from build123d import *

# Parameters (mm, degrees)
SKETCH1_W           = 100
SKETCH1_H           = 80
BOSS_EXTRUDE1_DEPTH = 4
SKETCH2_R           = 1
CUT_EXTRUDE1_DEPTH  = 65.156059729
BOSS_EXTRUDE2_DEPTH = 4
SKETCH4_R           = 1
CUT_EXTRUDE2_DEPTH  = 4
SKETCH5_R           = 1
CUT_EXTRUDE3_DEPTH  = 4
SKETCH6_R           = 6
CUT_EXTRUDE4_DEPTH  = 95.424573073
BOSS_EXTRUDE3_DEPTH = 4
SKETCH8_R           = 2.75
CUT_EXTRUDE5_DEPTH  = 308.949597178
CUT_EXTRUDE6_DEPTH  = 308.949597178
SKETCH11_R          = 1
SKETCH11_R_2        = 6
SKETCH11_W          = 15
SKETCH11_H          = 40
CUT_EXTRUDE7_DEPTH  = 4
SKETCH14_R          = 1
SKETCH14_R_2        = 6
BOSS_EXTRUDE5_DEPTH = 4
SKETCH15_R          = 6
CUT_EXTRUDE8_DEPTH  = 256.598728949
FILLET1_R           = 50


with BuildPart() as part:
    # Sketch1 → Boss-Extrude1 (new body)
    with BuildSketch(Plane(origin=(0, 0, 0), x_dir=(1, 0, 0), z_dir=(0, 1, 0))):
        Rectangle(SKETCH1_W, SKETCH1_H)
    extrude(amount=BOSS_EXTRUDE1_DEPTH)

    # Sketch2 → Cut-Extrude1 (cut, through all)
    with BuildSketch(Plane(origin=(0, 4, 0), x_dir=(1, 0, 0), z_dir=(0, 1, 0))):
        with Locations(Location((-40, 30, 0), (0, 0, 270))):
            Circle(SKETCH2_R)
        with Locations(Location((16.7, 30, 0), (0, 0, 270))):
            Circle(SKETCH2_R)
        with Locations(Location((16.7, -17.9, 0), (0, 0, 270))):
            Circle(SKETCH2_R)
        with Locations(Location((-40, -17.9, 0), (0, 0, 270))):
            Circle(SKETCH2_R)
    extrude(amount=-CUT_EXTRUDE1_DEPTH, mode=Mode.SUBTRACT)

    # Sketch3 → Boss-Extrude2 (add)
    with BuildSketch(Plane(origin=(0, 4, 0), x_dir=(1, 0, 0), z_dir=(0, 1, 0))):
        Polygon((7.993464363, -40), (50, -40), (50, -80), (-50, -80), (-50, -40), (-32.006535637, -40), (-32.006535637, -55), (7.993464363, -55), align=None)
    extrude(amount=-BOSS_EXTRUDE2_DEPTH)

    # Sketch4 → Cut-Extrude2 (cut)
    with BuildSketch(Plane(origin=(0, 4, 0), x_dir=(1, 0, 0), z_dir=(0, 1, 0))):
        with Locations(Location((-22.506535637, -61.25, 0), (0, 0, 270))):
            Circle(SKETCH4_R)
        with Locations(Location((-22.506535637, -73.75, 0), (0, 0, 270))):
            Circle(SKETCH4_R)
        with Locations(Location((-1.506535637, -73.75, 0), (0, 0, 270))):
            Circle(SKETCH4_R)
        with Locations(Location((-1.506535637, -61.25, 0), (0, 0, 270))):
            Circle(SKETCH4_R)
    extrude(amount=-CUT_EXTRUDE2_DEPTH, mode=Mode.SUBTRACT)

    # Sketch5 → Cut-Extrude3 (cut)
    with BuildSketch(Plane(origin=(0, 4, 0), x_dir=(1, 0, 0), z_dir=(0, 1, 0))):
        with Locations(Location((30, -45, 0), (0, 0, 270))):
            Circle(SKETCH5_R)
        with Locations(Location((30, -70, 0), (0, 0, 270))):
            Circle(SKETCH5_R)
    extrude(amount=-CUT_EXTRUDE3_DEPTH, mode=Mode.SUBTRACT)

    # Sketch6 → Cut-Extrude4 (cut, through all)
    with BuildSketch(Plane(origin=(0, 4, 0), x_dir=(1, 0, 0), z_dir=(0, 1, 0))):
        with Locations(Location((-12.006535637, -31, 0), (0, 0, 270))):
            Circle(SKETCH6_R)
    extrude(amount=-CUT_EXTRUDE4_DEPTH, mode=Mode.SUBTRACT)

    # Sketch7 → Boss-Extrude3 (add)
    with BuildSketch(Plane.XZ):
        with BuildLine():
            Line((-146.240473223, -40), (-50, -40))
            Line((-50, -40), (-50, 80))
            Line((-50, 80), (50, 80))
            Line((50, 80), (50, -40))
            Line((50, -40), (122.22740195, -40))
            ThreePointArc((122.22740195, -40), (148.208164063, -25), (148.208164063, 5))
            Line((148.208164063, 5), (13.974226477, 237.5))
            ThreePointArc((13.974226477, 237.5), (-12.006535637, 252.5), (-37.98729775, 237.5))
            Line((-37.98729775, 237.5), (-172.221235337, 5))
            ThreePointArc((-172.221235337, 5), (-172.221235337, -25), (-146.240473223, -40))
        make_face()
    extrude(amount=-BOSS_EXTRUDE3_DEPTH)

    # Sketch8 → Cut-Extrude5 (cut, through all)
    with BuildSketch(Plane.XZ):
        with Locations(Location((-27.006535637, -20.35, 0), (0, 0, 270))):
            Circle(SKETCH8_R)
        with Locations(Location((2.993464363, -20.35, 0), (0, 0, 270))):
            Circle(SKETCH8_R)
        with Locations(Location((-80.586867359, 124.415381057, 0), (0, 0, 90))):
            Circle(SKETCH8_R)
        with Locations(Location((-95.586867359, 98.434618943, 0), (0, 0, 90))):
            Circle(SKETCH8_R)
        with Locations(Location((71.573796086, 98.434618943, 0), (0, 0, 90))):
            Circle(SKETCH8_R)
        with Locations(Location((56.573796086, 124.415381057, 0), (0, 0, 90))):
            Circle(SKETCH8_R)
    extrude(amount=-CUT_EXTRUDE5_DEPTH, mode=Mode.SUBTRACT)

    # Sketch9 → Cut-Extrude6 (cut, through all)
    with BuildSketch(Plane(origin=(0, 4, 0), x_dir=(1, 0, 0), z_dir=(0, 1, 0))):
        with BuildLine():
            Line((32.993464363, -204.557713659), (-57.006535637, -204.557713659))
            Line((-57.006535637, -204.557713659), (-37.98729775, -237.5))
            ThreePointArc((-37.98729775, -237.5), (-12.006535637, -252.5), (13.974226477, -237.5))
            Line((13.974226477, -237.5), (32.993464363, -204.557713659))
        make_face()
        with BuildLine():
            Line((-172.221235337, -5), (-153.20199745, -37.942286341))
            Line((-153.20199745, -37.942286341), (-108.20199745, 40))
            Line((-108.20199745, 40), (-146.240473223, 40))
            ThreePointArc((-146.240473223, 40), (-172.221235337, 25), (-172.221235337, -5))
        make_face()
        with BuildLine():
            Line((122.22740195, 40), (84.188926177, 40))
            Line((84.188926177, 40), (129.188926177, -37.942286341))
            Line((129.188926177, -37.942286341), (148.208164063, -5))
            ThreePointArc((148.208164063, -5), (148.208164063, 25), (122.22740195, 40))
        make_face()
    extrude(amount=-CUT_EXTRUDE6_DEPTH, mode=Mode.SUBTRACT)

    # Sketch11 → Cut-Extrude7 (cut)
    with BuildSketch(Plane(origin=(0, 4, 0), x_dir=(1, 0, 0), z_dir=(0, 1, 0))):
        with Locations(Location((-109.506535637, -96.206535637, 0), (0, 0, 90))):
            Circle(SKETCH11_R)
        with Locations(Location((-109.506535637, -39.506535637, 0), (0, 0, 90))):
            Circle(SKETCH11_R)
        with Locations(Location((-61.606535637, -39.506535637, 0), (0, 0, 90))):
            Circle(SKETCH11_R)
        with Locations(Location((-61.606535637, -96.206535637, 0), (0, 0, 90))):
            Circle(SKETCH11_R)
        with Locations(Location((-34.506535637, -109.506535637, 0), (0, 0, 90))):
            Circle(SKETCH11_R)
        with Locations(Location((-9.506535637, -109.506535637, 0), (0, 0, 90))):
            Circle(SKETCH11_R)
        with Locations(Location((-5.756535637, -78, 0), (0, 0, 90))):
            Circle(SKETCH11_R)
        with Locations(Location((-18.256535637, -78, 0), (0, 0, 90))):
            Circle(SKETCH11_R)
        with Locations(Location((-18.256535637, -57, 0), (0, 0, 90))):
            Circle(SKETCH11_R)
        with Locations(Location((-5.756535637, -57, 0), (0, 0, 90))):
            Circle(SKETCH11_R)
        with Locations(Location((-48.506535637, -67.5, 0), (0, 0, 90))):
            Circle(SKETCH11_R_2)
        with Locations((-32.006535637, -67.5)):
            Rectangle(SKETCH11_W, SKETCH11_H)
    extrude(amount=-CUT_EXTRUDE7_DEPTH, mode=Mode.SUBTRACT)

    # Sketch14 → Boss-Extrude5 (add)
    with BuildSketch(Plane(origin=(0, 4, 0), x_dir=(1, 0, 0), z_dir=(0, 1, 0))):
        Polygon((-32.006535637, -47.5), (-24.506535637, -47.5), (-24.506535637, -55), (7.993464363, -55), (7.993464363, -40), (-32.006535637, -40), align=None)
        with Locations((-22.506535637, -61.25)):
            Circle(SKETCH14_R)
        with Locations((-1.506535637, -61.25)):
            Circle(SKETCH14_R)
        with Locations((-22.506535637, -73.75)):
            Circle(SKETCH14_R)
        with Locations((-1.506535637, -73.75)):
            Circle(SKETCH14_R)
        with Locations((30, -45)):
            Circle(SKETCH14_R)
        with Locations((30, -70)):
            Circle(SKETCH14_R)
        with Locations((-40, -17.9)):
            Circle(SKETCH14_R)
        with Locations((16.7, -17.9)):
            Circle(SKETCH14_R)
        with Locations((-40, 30)):
            Circle(SKETCH14_R)
        with Locations((16.7, 30)):
            Circle(SKETCH14_R)
        with Locations((-12.006535637, -31)):
            Circle(SKETCH14_R_2)
    extrude(amount=-BOSS_EXTRUDE5_DEPTH)

    # Sketch15 → Cut-Extrude8 (cut, through all)
    with BuildSketch(Plane(origin=(0, 4, 0), x_dir=(1, 0, 0), z_dir=(0, 1, 0))):
        with Locations(Location((-48.506535637, -67.5, 0), (0, 0, 90))):
            Circle(SKETCH15_R)
        with Locations(Location((6.243464363, -99.109927238, 0), (0, 0, 270))):
            Circle(SKETCH15_R)
        with Locations(Location((6.243464363, -35.890072762, 0), (0, 0, 270))):
            Circle(SKETCH15_R)
    extrude(amount=-CUT_EXTRUDE8_DEPTH, mode=Mode.SUBTRACT)

    # Fillet1
    fillet1_edges = [part.edges().sort_by_distance(p)[0] for p in [
        (32.993464363, 2, 204.557713659),
        (-57.006535637, 2, 204.557713659),
        (-153.20199745, 2, 37.942286341),
        (-108.20199745, 2, -40),
        (84.188926177, 2, -40),
        (129.188926177, 2, 37.942286341),
    ]]
    fillet(fillet1_edges, radius=FILLET1_R)


solid = part.part
Model file for the job. Use its own axes, mm. Give positions to 0.01 mm unless a question says otherwise; leave off trailing zeros. Loops run counter-clockwise (first coordinate to the right, second up) from the corner with the lowest first, then second, coordinate; pieces in that order, holes last.
Item 1: Slice it at C-C (z = 4). Write the cut outline in (x, y), plus the area to 3 significant figures.
Check values:
outline: (-133.61, 0) - (109.59, 0) - (109.59, 4) - (-133.61, 4) - close
area: 973 mm2
Item 2: Slice it at B-B (y = 1.55). Give the number of separate pieces and of enclosed holes in the cut face, plus the area to 3 significant figures.
Check values:
separate pieces: 1
enclosed holes: 20
area: 47,600 mm2
Item 3: Mould opens along X. For faces 1 (the face through (3.945, 2.028, 41.433)), 2 (the face through (81.562, 1.972, 120.434)), 3 (the face through (-14, 4, 53)), 4 (the face through (-29.446, 1.972, -21.619)) say: +X half, -X half, draft (parallel to the pull), parting line (faces both ways), or undercut.
Check values:
face 1: undercut
face 2: +X half
face 3: draft
face 4: undercut
Item 4: Drill centre lines: line 1 along X through (y, z) = (1.3, -22); line 2 along Z through (x, y) = (1, 2.8); line 3 along X through (y, z) = (2.75, 77.5). Where is each one in solid material? Low to high.
Check values:
line 1: x = -117.75 to -29.21, -24.81 to 0.79, 5.19 to 93.74
line 2: z = -40 to -22.24, -18.46 to 32.97, 38.81 to 96.19, 102.03 to 204.56
line 3: x = -130.36 to -39.51, -24.51 to -19.12, -17.39 to -6.62, -4.89 to 106.35
Item 5: Slice it at A-A (z = 67.5). Write the cut outline in (x, y).
Check values:
outline: (-136.14, 0) - (-54.51, 0) - (-54.51, 4) - (-136.14, 4) - close; (-42.51, 0) - (-39.51, 0) - (-39.51, 4) - (-42.51, 4) - close; (-24.51, 0) - (112.12, 0) - (112.12, 4) - (-24.51, 4) - close
Item 6: Drop flat-ended pins along their axis: P1, Ø2.5, axis at x = -109.51, z = 39.51, coming from the +Y side; P2, Ø1.2, axis at y = 1.5, z = 74, coming from the +X side; P3, Ø2, axis at y = 2.5, z = 71.5, coming from the -X side; P4, Ø11, axis at x = 6.24, z = 99.11, coming from the +Y side. Give the stop position or say it passes through.
Check values:
P1: stops at y = 4
P2: stops at x = 108.72
P3: stops at x = -134.4
P4: passes through
